Work out the finished part from the listing and answer in its coordinate system (mm). Face numbers are marked on the shaded views. Give positions to 0.01 mm unless a question says otherwise; leave off trailing zeros. Write each loop counter-clockwise with the first axis right and the second up, starting at its lowest first coordinate (ties: lowest second). Pieces come first, ordered by that corner, then holes.
1) Straight lines are drawn through the part: probe 1 along Y at (x, z) = (0, 4.75); probe 2 along Y at (x, z) = (0, 8.5); probe 3 along X at (y, z) = (-6, 4). For each, find the intervals that lie inside material, in ascending order.
2) Find section C-C (z = 3). Determine the outline of the cut face in (x, y).
3) Given pin 1 Ø5 at (y, z) = (17.5, 2.5) entering from -X; pin 2 Ø8 at (y, z) = (19, 13) entering from -X; pin 3 Ø5 at (x, y) = (13.5, -5.5) entering from -Z; pin 4 Ø8 at (x, z) = (-5, 4.5) entering from +Y, each flat-ended and moving along its own axis, determine where each tip first touches the part or whether it passes through.
4) Determine the mould class of the marked faces 1, 2 and 3 for opening direction Y: pulls with the +Y half, pulls with the -Y half, needs draft (parallel to the pull), parting line crosses it, or undercut.
5) Find section D-D (z = 7). Determine the outline of the cut face in (x, y), plus the area to 3 significant figures.
6) Find section A-A (x = 0). Determine the outline of the cut face in (y, z).
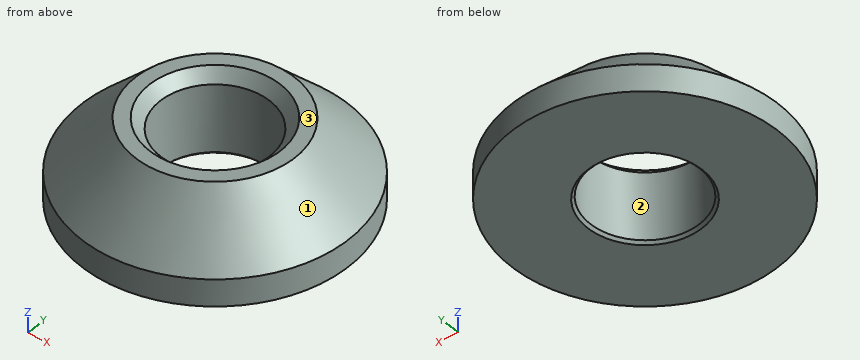
Autodesk Inventor part; units mm, degrees
ref_plane "YZ Plane" through (0, 0, 0) normal (1, 0, 0) x (0, 1, 0)
ref_plane "XZ Plane" through (0, 0, 0) normal (0, 1, 0) x (-1, 0, 0)
ref_plane "XY Plane" through (0, 0, 0) normal (0, 0, 1) x (1, 0, 0)
sketch "Sketch1" plane through (0, 0, 0) normal (0, 0, 1) x (1, 0, 0)
  circle A0 centre (0, 0) radius 24.75
  dimension "d0" = 49.5
extrude "Extrusion1" add sketch "Sketch1" along normal blind 15
sketch "Sketch2" plane through (0, 0, 15) normal (0, 0, 1) x (1, 0, 0)
  circle A0 centre (0, 0) radius 24.75
hole "Hole1" at (0, 0, 15) direction (0, 0, -1) diameter 20.269 depth 15 tip angle 118
chamfer "Chamfer1" distance 10 angle 45 1 edges at (-24.75, 0, 15)
chamfer "Chamfer2" distance 2 angle 45 1 edges at (0, 10.1345, 15)
chamfer "Chamfer3" distance 0.5 angle 45 1 edges at (0, 10.1345, 0)
properties part number "LUVA(24)" material "Carbon Steel"
Results:
1. probe 1: y = -24.75 to -10.13, 10.13 to 24.75
1. probe 2: y = -21.25 to -10.13, 10.13 to 21.25
1. probe 3: x = -24.01 to -8.17, 8.17 to 24.01
2. outline: circle Ø49.5 at (0, 0); hole circle Ø20.27 at (0, 0)
3. pin 1: stops at x = -19.69
3. pin 2: stops at x = -11.08
3. pin 3: stops at z = 0
3. pin 4: stops at y = 24.73
4. face 1: parting line crosses it
4. face 2: undercut
4. face 3: needs draft
5. outline: circle Ø45.5 at (0, 0); hole circle Ø20.27 at (0, 0)
5. area: 1,300 mm2
6. outline: (-24.75, 0) - (-10.63, 0) - (-10.13, 0.5) - (-10.13, 13) - (-12.13, 15) - (-14.75, 15) - (-24.75, 5) - close; (10.13, 0.5) - (10.63, 0) - (24.75, 0) - (24.75, 5) - (14.75, 15) - (12.13, 15) - (10.13, 13) - close
